Autodesk Inventor part; units mm, degrees
ref_plane "YZ Plane" through (0, 0, 0) normal (1, 0, 0) x (0, 1, 0)
ref_plane "XZ Plane" through (0, 0, 0) normal (0, 1, 0) x (-1, 0, 0)
ref_plane "XY Plane" through (0, 0, 0) normal (0, 0, 1) x (1, 0, 0)
sketch "Sketch1" plane through (0, 0, 0) normal (0, 1, 0) x (-1, 0, 0)
  circle A0 centre (0, 0) radius 1.75
  circle A1 centre (0, 0) radius 3.5
  dimension "d0" = 3.5
  dimension "d1" = 7
extrude "Extrusion1" add sketch "Sketch1" along normal blind 0.5
chamfer "Chamfer1" distance 0.1 angle 45 2 edges at (1.75, 0, 0) (1.75, 0.5, 0)
fillet "Fillet1" radius 0.1 2 edges at (3.5, 0.5, 0) (3.5, 0, 0)
properties part number "M3 Screw Washer" material "Stainless Steel"
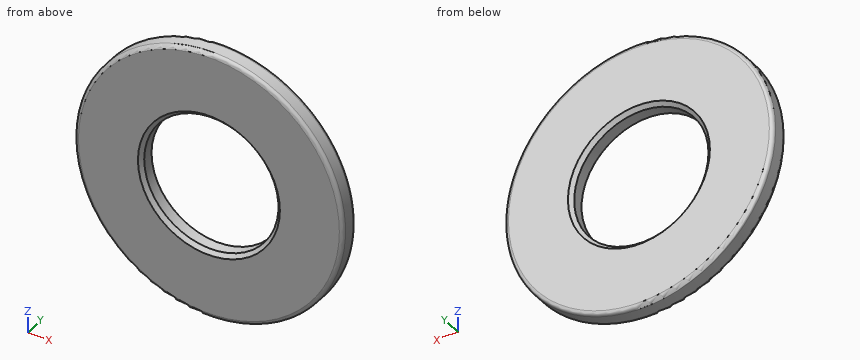
The listing builds one solid part. Answer for the finished solid, in the listing's coordinates (mm). Coordinates: 2 decimals unless noted, no trailing zeros. Loops run counter-clockwise (first coordinate to the right, second up) from the corner with the lowest first, then second, coordinate; pieces in that order, holes last. Notation, with made-up numbers: (9.5, 42.5) - (48.5, 42.5) arc R30 cw to (48.5, 69.5) - close; hole circle Ø3 at (52, 69). An arc over 180 degrees is marked (long way). Use a Markdown table: item, result. Add a question column.
1) The part is cut by section A-A, the plane x = 0. Give the vertices of the cut face in (y, z), and give its area (3 significant figures).
2) The part is cut by section C-C, the plane y = 0.3. Give the vertices of the cut face in (x, z).
3) Find the intervals of material crossed by line 1 (Z direction, x = 0, y = 0.35); line 2 (Z direction, x = 1.5, y = 0.3); line 3 (X direction, y = 0.1, z = 2), in increasing order.
4) The part is cut by section B-B, the plane z = 0. Give the vertices of the cut face in (x, y), and give its area (3 significant figures).
Here are the results:
| question | item | result |
|---|---|---|
| 1 | outline | (0, -3.4) arc R0.1 ccw to (0.1, -3.5) - (0.4, -3.5) arc R0.1 ccw to (0.5, -3.4) - (0.5, -1.85) - (0.4, -1.75) - (0.1, -1.75) - (0, -1.85) - close; (0, 1.85) - (0.1, 1.75) - (0.4, 1.75) - (0.5, 1.85) - (0.5, 3.4) arc R0.1 ccw to (0.4, 3.5) - (0.1, 3.5) arc R0.1 ccw to (0, 3.4) - close |
| 1 | area | 1.72 mm^2 |
| 2 | outline | circle Ø7 at (0, 0); hole circle Ø3.5 at (0, 0) |
| 3 | line 1 | z = -3.5 to -1.75, 1.75 to 3.5 |
| 3 | line 2 | z = -3.16 to -0.9, 0.9 to 3.16 |
| 3 | line 3 | x = -2.87 to 2.87 |
| 4 | outline | (-3.5, 0.1) arc R0.1 ccw to (-3.4, 0) - (-1.85, 0) - (-1.75, 0.1) - (-1.75, 0.4) - (-1.85, 0.5) - (-3.4, 0.5) arc R0.1 ccw to (-3.5, 0.4) - close; (1.75, 0.1) - (1.85, 0) - (3.4, 0) arc R0.1 ccw to (3.5, 0.1) - (3.5, 0.4) arc R0.1 ccw to (3.4, 0.5) - (1.85, 0.5) - (1.75, 0.4) - close |
| 4 | area | 1.72 mm^2 |
